Autodesk Inventor part; units mm, degrees
ref_plane "YZ Plane" through (0, 0, 0) normal (1, 0, 0) x (0, 1, 0)
ref_plane "XZ Plane" through (0, 0, 0) normal (0, 1, 0) x (-1, 0, 0)
ref_plane "XY Plane" through (0, 0, 0) normal (0, 0, 1) x (1, 0, 0)
sketch "Esquisse1" plane through (0, 0, 0) normal (0, 1, 0) x (-1, 0, 0)
  line L0 (0, 0) -> (0, 2.45)
  line L1 (0, 0) -> (2.45, 0) construction
  line L2 (0, 2.45) -> (28, 2.45)
  line L3 (28, 2.45) -> (28, 22.55)
  line L4 (28, 22.55) -> (-28, 22.55)
  line L5 (-28, 22.55) -> (-28, 2.45)
  line L6 (-28, 2.45) -> (0, 2.45)
  line L7 (0, 0) -> (30, 0)
  line L8 (30, 0) -> (30, 25)
  line L9 (30, 25) -> (-30, 25)
  line L10 (-30, 25) -> (-30, 0)
  line L11 (-30, 0) -> (0, 0)
  dimension "d0" = 2.45
  dimension "d1" = 90
  dimension "d2" = 28
  dimension "d3" = 20.1
  dimension "d4" = 56
  dimension "d5" = 30
  dimension "d6" = 25
  dimension "d7" = 60
extrude "Extrusion1" add sketch "Esquisse1" along normal blind 27
sketch "Esquisse2" plane through (30, 0, 0) normal (0, 0, -1) x (-1, 0, 0)
  line L0 (30, 0) -> (30, 27)
  line L1 (60, 27) -> (0, 27)
  line L2 (0, 0) -> (0, 27)
  line L3 (0, 13.5) -> (60, 13.5)
  line L4 (60, 0) -> (60, 27)
  circle A0 centre (30, 13.5) radius 8
  circle A1 centre (30, 13.5) radius 9
  dimension "d10" = 16
  dimension "d11" = 18
extrude "Extrusion2" add sketch "Esquisse2" along normal blind 10 contours A1 L3 A0 L0 | L0 A0 L3 A1 | A1 L0 A0 L3 | L3 A0 L0 A1
sketch "Esquisse3" plane through (0, 0, 0) normal (0, 1, 0) x (-1, 0, 0)
  line L0 (-9, -10) -> (9, -10)
  line L1 (0, -10) -> (0, -5)
  point P0 (0, 0)
  dimension "d14" = 5
hole "Perçage1" at (0, 0, -5) direction (0, 1, 0) diameter 4 end through all
sketch "Esquisse7" plane through (0, 0, 0) normal (0, -1, 0) x (1, 0, 0)
  line L0 (-30, 0) -> (-30, 25)
  line L1 (30, 0) -> (-30, 0)
  line L2 (30, 25) -> (30, 0)
  line L3 (-30, 25) -> (30, 25)
  line L4 (28, 22.55) -> (-28, 22.55)
  line L5 (-28, 2.45) -> (28, 2.45)
  line L6 (-28, 22.55) -> (-28, 2.45)
  line L7 (28, 2.45) -> (28, 22.55)
  point P0 (0, 0)
extrude "Extrusion5" add sketch "Esquisse7" along normal blind 13.14
sketch "Esquisse11" plane through (0, -13.14, 0) normal (0, -1, 0) x (1, 0, 0)
  line L0 (28, 22.55) -> (28, 2.45)
  line L1 (-28, 22.55) -> (28, 22.55)
  line L2 (28, 2.45) -> (28, 22.55)
  line L3 (28, 22.55) -> (28, 2.45)
  line L4 (28, 22.55) -> (-28, 22.55)
  line L5 (28, 22.55) -> (22, 22.55)
  line L6 (22, 22.55) -> (22, 2.45)
  line L7 (22, 2.45) -> (28, 2.45)
  line L8 (-28, 22.55) -> (-22, 22.55)
  line L9 (-22, 22.55) -> (-22, 2.45)
  line L10 (-28, 2.45) -> (28, 2.45)
  line L11 (-22, 2.45) -> (-28, 2.45)
  line L12 (-28, 22.55) -> (-28, 2.45)
  line L13 (-28, 22.55) -> (-28, 2.45)
  point P0 (0, 0)
  dimension "d46" = 6
  dimension "d47" = 6
extrude "Extrusion6" add sketch "Esquisse11" against normal blind 9 contours L0 L7 L6 L1 | L9 L10 L12 L1
sketch "Esquisse12" plane through (0, -4.14, 0) normal (0, 1, 0) x (1, 0, 0)
  line L0 (-22, -22.55) -> (-28, -22.55)
  line L1 (-28, -22.55) -> (-28, -13.5)
  line L2 (-28, -22.55) -> (-28, -2.45)
  line L3 (-28, -13.5) -> (-22, -13.5)
  line L4 (-22, -22.55) -> (-22, -2.45)
  line L5 (-22, -13.5) -> (-22, -11.5)
  line L6 (-22, -11.5) -> (-28, -11.5)
  line L7 (-28, -13.5) -> (-28, -11.5)
  line L8 (-28, -11.5) -> (-28, -13.5)
  line L9 (28, -2.45) -> (28, -22.55)
  line L10 (28, -22.55) -> (28, -13.5)
  line L11 (28, -13.5) -> (22, -13.5)
  line L12 (22, -13.5) -> (22, -11.5)
  line L13 (22, -22.55) -> (22, -2.45)
  line L14 (22, -11.5) -> (28, -11.5)
  line L15 (28, -11.5) -> (28, -13.5)
  line L16 (28, -13.5) -> (28, -11.5)
  point P0 (0, 0)
  dimension "d50" = 9.05
  dimension "d51" = 2
  dimension "d52" = 6
extrude "Extrusion7" cut sketch "Esquisse12" against normal blind 2 contours L3 L2 L6 L4 | L9 L11 L12 L14
sketch "Esquisse13" plane through (0, -4.14, 0) normal (0, 1, 0) x (1, 0, 0)
  line L0 (-28, -22.55) -> (-28, -2.45)
  line L1 (-28, -22.55) -> (-28, -12.5)
  line L2 (-28, -2.45) -> (-22, -2.45)
  line L3 (-28, -12.5) -> (-25, -12.5)
  line L4 (-25, -12.5) -> (-25, -7.5)
  line L5 (-25, -12.5) -> (-25, -17.5)
  line L6 (28, -13.5) -> (28, -22.55)
  line L7 (28, -22.55) -> (28, -12.5)
  line L8 (28, -12.5) -> (25, -12.5)
  line L9 (25, -12.5) -> (25, -7.5)
  line L10 (25, -7.5) -> (25, -17.5)
  point P0 (0, 0)
  dimension "d55" = 10.05
  dimension "d56" = 3
  dimension "d57" = 5
  dimension "d58" = 5
  dimension "d59" = 3
  dimension "d60" = 5
  dimension "d61" = 10
hole "Perçage3" at (-25, -4.14, 17.5) at (-25, -4.14, 7.5) at (25, -4.14, 17.5) at (25, -4.14, 7.5) direction (0, -1, 0) diameter 3.242 depth 11.8 tip angle 118
sketch "Esquisse14" plane through (30, 27, 25) normal (1, 0, 0) x (0, 0, -1)
  line L0 (0, -40.14) -> (0, 0)
  line L1 (0, 0) -> (2.45, 0)
  line L2 (0, 0) -> (25, 0)
  line L3 (2.45, 0) -> (2.45, -13.14)
  line L4 (2.45, -31.14) -> (2.45, -40.14)
  line L5 (2.45, -13.14) -> (22.55, -13.14)
  line L6 (22.55, -13.14) -> (22.55, 0)
  line L7 (2.45, 0) -> (22.55, 0)
  line L8 (25, -40.14) -> (25, 0)
  point P0 (25, -27)
  dimension "d69" = 2.45
  dimension "d70" = 13.14
  dimension "d71" = 20.1
extrude "Extrusion8" cut sketch "Esquisse14" against normal through all
properties part number "Attache servomoteur_bogie"
Design review of the part built by this model. Coordinates are the model's own, in mm. A direction names the side the tool comes from. Give positions to 0.01 mm unless a question says otherwise; leave off trailing zeros. Write each loop counter-clockwise with the first axis right and the second up, starting at its lowest first coordinate (ties: lowest second). Pieces come first, ordered by that corner, then holes.
(1) Add section A-A (z = 7.5). Give the boundary of the cut face in (x, y), and give its area (3 significant figures).
Checked values:
outline: (-30, -13.14) - (-26.62, -13.14) - (-26.62, -4.14) - (-28, -4.14) - (-28, 13.86) - (-30, 13.86) - close; (-23.38, -13.14) - (-22, -13.14) - (-22, -4.14) - (-23.38, -4.14) - close; (22, -13.14) - (23.38, -13.14) - (23.38, -4.14) - (22, -4.14) - close; (26.62, -13.14) - (30, -13.14) - (30, 13.86) - (28, 13.86) - (28, -4.14) - (26.62, -4.14) - close
area: 158 mm2
(2) Add section C-C (x = -20). Give the boundary of the cut face in (y, z).
Checked values:
outline: (-13.14, 0) - (27, 0) - (27, 2.45) - (-13.14, 2.45) - close; (-13.14, 22.55) - (27, 22.55) - (27, 25) - (-13.14, 25) - close
(3) Clearance check with flat-ended pins moving along their axes: pin 1 Ø5 at (x, y) = (-3, 15.5) entering from -Z; pin 2 Ø5 at (x, z) = (-25, 6) entering from +Y; pin 3 Ø6.5 at (x, z) = (0, -5) entering from -Y; pin 4 Ø6 at (x, z) = (13.5, -3.5) entering from +Y. State where each tip first meets the part, or that it passes through.
Checked values:
pin 1: stops at z = 0
pin 2: stops at y = -4.14
pin 3: stops at y = 4.5
pin 4: passes through
(4) Mouldability with a two-part tool opening along X and no side actions: class faces 4 (the face through (-4.153, 21.485, -4.93)), 5 (the face through (30, 3, 13)), 6 (the face through (22, -9, 13)), 7 (the face through (29, 13.86, 13)) as +X half, -X half, draft (parallel to the pull), parting line (faces both ways), or undercut.
Checked values:
face 4: parting line
face 5: +X half
face 6: undercut
face 7: draft
(5) Wall thickness on line 1 along Z through (x, y) = (25, -5.75); line 2 along Z through (x, y) = (25, -6.5); line 3 along Z through (x, y) = (-2, -6): over which ranges is each line inside the solid? List them lowest first.
Checked values:
line 1: z = 0 to 5.88, 9.12 to 11.5, 13.5 to 15.88, 19.12 to 25
line 2: z = 0 to 5.88, 9.12 to 15.88, 19.12 to 25
line 3: z = 0 to 2.45, 22.55 to 25
(6) Tool access review of faces 1 (the face through (0, -13.14, 2)), 2 (the face through (-25, -5, 13.5)), 3 (the face through (0, 13, 0)): name each direction out of +Z, -Z, +X, -X, +Y, -Y from which nothing blocks a thin tool from reaching the whole face with its end or side.
Checked values:
face 1: +Z, -Z, +X, -X, -Y
face 2: +Y
face 3: -Z
(7) Add section D-D (z = 3.5). Give the boundary of the cut face in (x, y), and give its area (3 significant figures).
Checked values:
outline: (-30, -13.14) - (-22, -13.14) - (-22, -4.14) - (-28, -4.14) - (-28, 13.86) - (-30, 13.86) - close; (22, -13.14) - (30, -13.14) - (30, 13.86) - (28, 13.86) - (28, -4.14) - (22, -4.14) - close
area: 216 mm2
(8) Add section B-B (y = -5). Give the boundary of the cut face in (x, z), and give its area (3 significant figures).
Checked values:
outline: (-30, 0) - (30, 0) - (30, 25) - (-30, 25) - close; hole (-28, 11.5) - (-22, 11.5) - (-22, 2.45) - (22, 2.45) - (22, 11.5) - (28, 11.5) - (28, 13.5) - (22, 13.5) - (22, 22.55) - (-22, 22.55) - (-22, 13.5) - (-28, 13.5) - close; hole circle Ø3.24 at (-25, 7.5); hole circle Ø3.24 at (-25, 17.5); hole circle Ø3.24 at (25, 7.5); hole circle Ø3.24 at (25, 17.5)
area: 559 mm2
